Part model, mm, in its own coordinate system. A direction names the side the tool comes from. Round coordinates to 2 decimals unless told otherwise and drop trailing zeros. Loops run counter-clockwise (first coordinate to the right, second up) from the corner with the lowest first, then second, coordinate; pieces in that order, holes last. Notation, with made-up numbers: (56, 84.5) -> (70, 84.5) arc R18 ccw to (70, 103.5) -> close; hole circle Ø7 at (9.5, 31). An arc over 180 degrees is marked (long way). Use a Markdown table: item, result. Add a question column.
Item 1: Flat gauge pins, fed straight in: pin 1 (5 mm diameter, centred on x = 6, z = -16.5, fed in from -Y); pin 2 (1.4 mm diameter, centred on x = 22, y = 1.5, fed in from +Z); pin 3 (2.5 mm diameter, centred on x = -25, y = 2.5, fed in from +Z). Where does each tip first touch, or does it go through?
Item 2: Probe line 1 (X direction, y = 1.9, z = -20) (3 decimals); line 2 (Z direction, x = 19.5, y = 1.9); line 3 (X direction, y = 4.4, z = -16). List the from-to ranges inside material, lowest first. Write a range as [from, to].
Item 3: Cut at B-B, the plane z = -20. List the corners of the cut face in (x, y) (3 decimals).
Item 4: Cut at D-D, the plane y = 1.35. State how many separate pieces and enclosed holes the cut face has, plus the area to 3 significant figures.
Item 5: Which spindle directions (+Z, -Z, +X, -X, +Y, -Y) get a long thin tool onto all of the face, cutting with end or side? Do faces 1 (the face through (19, 3, -1)), 2 (the face through (22.875, 3, -2)), 3 (the face through (18.625, 3, -4)). Say none if no direction does.
Item 6: Two-plate mould, pull along X, no slides. Class faces 4 (the face through (-19, 3, -1)), 5 (the face through (-17.5, 2, 8)), 6 (the face through (8, 3, -18)): pulls with the +X half, pulls with the -X half, needs draft (parallel to the pull), parting line crosses it, or undercut.
Item 7: Cut at C-C, the plane x = 14. List the corners of the cut face in (y, z).
Item 8: Cut at A-A, the plane z = 0. List the corners of the cut face in (x, y).
```python
from build123d import *

# Parameters (mm, degrees)
ESQUISSE1_W             = 35
ESQUISSE1_H             = 35
BOSS_EXTRU_1_DEPTH      = 5
ESQUISSE3_R             = 15
ENL_V_MAT_EXTRU_1_DEPTH = 5
ESQUISSE5_W             = 10
ESQUISSE5_H             = 16.5
BOSS_EXTRU_3_DEPTH      = 5
ENL_V_MAT_EXTRU_3_DEPTH = 10
ESQUISSE2_W             = 55
ESQUISSE2_H             = 5
BOSS_EXTRU_4_DEPTH      = 5
ESQUISSE8_W             = 16
ESQUISSE8_H             = 9.81142246
ENL_V_MAT_EXTRU_5_DEPTH = 5
ESQUISSE9_W             = 5
ESQUISSE9_H             = 5
ENL_V_MAT_EXTRU_6_DEPTH = 5
ESQUISSE10_R            = 1.5
ENL_V_MAT_EXTRU_7_DEPTH = 6


with BuildPart() as part:
    # Esquisse1 → Boss.-Extru.1 (new body)
    with BuildSketch(Plane(origin=(0, 0, 0), x_dir=(1, 0, 0), z_dir=(0, 1, 0))):
        Rectangle(ESQUISSE1_W, ESQUISSE1_H)
    extrude(amount=BOSS_EXTRU_1_DEPTH)

    # Esquisse3 → Enlèv. mat.-Extru.1 (cut)
    with BuildSketch(Plane(origin=(0, 5, 0), x_dir=(1, 0, 0), z_dir=(0, 1, 0))):
        Circle(ESQUISSE3_R)
    extrude(amount=-ENL_V_MAT_EXTRU_1_DEPTH, mode=Mode.SUBTRACT)

    # Esquisse5 → Boss.-Extru.3 (add)
    with BuildSketch(Plane(origin=(0, 5, 0), x_dir=(1, 0, 0), z_dir=(0, 1, 0))):
        with Locations((-22.5, 9.25)):
            Rectangle(ESQUISSE5_W, ESQUISSE5_H)
    boss_extru_3 = extrude(amount=-BOSS_EXTRU_3_DEPTH)

    # Symétrie1: Boss.-Extru.3 across plane
    add(boss_extru_3.mirror(Plane(origin=(0, 0, 0), x_dir=(0, 0, 1), z_dir=(1, 0, 0))))

    # Esquisse7 → Enlèv. mat.-Extru.3 (cut)
    with BuildSketch(Plane(origin=(0, 5, 0), x_dir=(1, 0, 0), z_dir=(0, 1, 0))):
        Polygon((-22.875, 1), (-22.875, 2.75), (-24.375, 2.75), (-24.375, 5.5), (-22.875, 5.5), (-22.875, 7), (-20.125, 7), (-20.125, 5.5), (-18.625, 5.5), (-18.625, 2.75), (-20.125, 2.75), (-20.125, 1), align=None)
    enl_v_mat_extru_3 = extrude(amount=-ENL_V_MAT_EXTRU_3_DEPTH, mode=Mode.SUBTRACT)

    # Symétrie2: Enlèv. mat.-Extru.3 across plane
    add(enl_v_mat_extru_3.mirror(Plane(origin=(0, 0, 0), x_dir=(0, 0, 1), z_dir=(1, 0, 0))), mode=Mode.SUBTRACT)

    # Esquisse2 → Boss.-Extru.4 (add)
    with BuildSketch(Plane(origin=(0, 5, 0), x_dir=(1, 0, 0), z_dir=(0, 1, 0))):
        with Locations((0, 20)):
            Rectangle(ESQUISSE2_W, ESQUISSE2_H)
    extrude(amount=-BOSS_EXTRU_4_DEPTH)

    # Esquisse8 → Enlèv. mat.-Extru.5 (cut)
    with BuildSketch(Plane(origin=(0, 5, 0), x_dir=(1, 0, 0), z_dir=(0, 1, 0))):
        with Locations((0, 17.59428877)):
            Rectangle(ESQUISSE8_W, ESQUISSE8_H)
    extrude(amount=-ENL_V_MAT_EXTRU_5_DEPTH, mode=Mode.SUBTRACT)

    # Esquisse9 → Enlèv. mat.-Extru.6 (cut)
    with BuildSketch(Plane(origin=(0, 5, 0), x_dir=(1, 0, 0), z_dir=(0, 1, 0))):
        with Locations((-20, 20)):
            Rectangle(ESQUISSE9_W, ESQUISSE9_H)
        with Locations((20, 20)):
            Rectangle(ESQUISSE9_W, ESQUISSE9_H)
    extrude(amount=-ENL_V_MAT_EXTRU_6_DEPTH, mode=Mode.SUBTRACT)

    # Esquisse10 → Enlèv. mat.-Extru.7 (cut, through all)
    with BuildSketch(Plane(origin=(0, 5, 0), x_dir=(1, 0, 0), z_dir=(0, 1, 0))):
        with Locations((-13.625, 20)):
            Circle(ESQUISSE10_R)
        with Locations((13.625, 20)):
            Circle(ESQUISSE10_R)
    extrude(amount=-ENL_V_MAT_EXTRU_7_DEPTH, mode=Mode.SUBTRACT)


solid = part.part
```
A:
| question | item | result |
|---|---|---|
| 1 | pin 1 | stops at y = 0 |
| 1 | pin 2 | stops at z = -7 |
| 1 | pin 3 | stops at z = -1 |
| 2 | line 1 | x = [-27.5, -22.5], [-17.5, -15.125], [-12.125, -8], [8, 12.125], [15.125, 17.5], [22.5, 27.5] |
| 2 | line 2 | z = [-17.5, -5.5], [-2.75, -1] |
| 2 | line 3 | x = [-27.5, -8], [8, 27.5] |
| 3 | outline | (-27.5, 0) -> (-22.5, 0) -> (-22.5, 5) -> (-27.5, 5) -> close; (-17.5, 0) -> (-15.125, 0) -> (-15.125, 5) -> (-17.5, 5) -> close; (-12.125, 0) -> (-8, 0) -> (-8, 5) -> (-12.125, 5) -> close; (8, 0) -> (12.125, 0) -> (12.125, 5) -> (8, 5) -> close; (15.125, 0) -> (17.5, 0) -> (17.5, 5) -> (15.125, 5) -> close; (22.5, 0) -> (27.5, 0) -> (27.5, 5) -> (22.5, 5) -> close |
| 4 | separate pieces | 1 |
| 4 | enclosed holes | 2 |
| 4 | area | 878 mm^2 |
| 5 | face 1 | +Z, +X, +Y, -Y |
| 5 | face 2 | +Z, +Y, -Y |
| 5 | face 3 | +Y, -Y |
| 6 | face 4 | needs draft |
| 6 | face 5 | pulls with the -X half |
| 6 | face 6 | undercut |
| 7 | outline | (0, -22.5) -> (5, -22.5) -> (5, -21.45) -> (0, -21.45) -> close; (0, -18.55) -> (5, -18.55) -> (5, -5.39) -> (0, -5.39) -> close; (0, 5.39) -> (5, 5.39) -> (5, 17.5) -> (0, 17.5) -> close |
| 8 | outline | (-17.5, 0) -> (-15, 0) -> (-15, 5) -> (-17.5, 5) -> close; (15, 0) -> (17.5, 0) -> (17.5, 5) -> (15, 5) -> close |
